Here's how the part is built. I have some questions about the finished solid (model axes, mm). A direction names the side the tool comes from. Round coordinates to 2 decimals unless told otherwise and drop trailing zeros. Write each loop counter-clockwise with the first axis right and the second up, starting at its lowest first coordinate (ties: lowest second). Pieces come first, ordered by that corner, then holes. Notation, with made-up numbers: (-30.75, -32.75) - (-12.75, -32.75) arc R6 cw to (-12.75, -21.75) - close; hole circle Ø5 at (75, -25). An arc over 180 degrees is marked (long way). Write item = value, one per line. Start each with the question number.
Item 1: If I drill on line 1 along Z through (x, y) = (54.75, -17.5); line 2 along Z through (x, y) = (-65, -22); line 3 along X through (y, z) = (-39.5, 45), over which ranges is the centre line in solid material (lowest first)? Write a range as [from, to].
Item 2: Which directions (+Z, -Z, +X, -X, +Y, -Y) give clear straight access to the entire face, cutting with the end or side of a thin tool? Please do faces 1 (the face through (-9.764, -44.614, 74.362)), 2 (the face through (79.26, -7.96, 23)), 3 (the face through (65.651, -17.745, 60.043)).
Item 3: Thinking about a two-plate mould opening in Y: for faces 4 (the face through (-1, 0, 1)), 5 (the face through (-75.72, -17.74, -75.49)), 6 (the face through (69.38, -18.58, 15.12)), which applies, pulls with the +Y half, pulls with the -Y half, needs draft (parallel to the pull), parting line crosses it, or undercut?
Item 4: For P1, Ø1, axis at y = -46, z = 43.5, coming from the -X side; P2, Ø16, axis at y = -17.5, z = 20, coming from the +X side; P3, Ø3, axis at x = 60, z = -55.5, coming from the -Y side, each with a flat end and sliding along its axis, tell me the tip position at first contact or that it passes through.
Item 5: If we section it at A-A (y = -51.5): Please give me the cut outline in (x, z).
```python
from build123d import *

# Parameters (mm, degrees)
F0_W      = 160
F0_H      = 160
F0_R      = 75
F1_DEPTH  = 35
F2_DEPTH  = 57.5
F3_SIZE2  = 3
F3_SIZE   = 3
F4_R      = 15
F5_D      = 10
F7_D      = 8
F7_DEPTH  = 40
F8_R      = 4
F9_DEPTH  = 34.5
F8_R_2    = 5
F10_DEPTH = 20
F8_R_3    = 10
F11_DEPTH = 1.5


with BuildPart() as f1:
    # F0 (on Front) → F1 (new body)
    with BuildSketch(Plane.XZ):
        Rectangle(F0_W, F0_H)
        Circle(F0_R, mode=Mode.SUBTRACT)
        Circle(F0_R)
    extrude(amount=F1_DEPTH)

    # F0 (on Front) → F2 (join)
    with BuildSketch(Plane.XZ):
        Circle(F0_R)
    extrude(amount=F2_DEPTH)

    # F3
    f3_edges = [f1.edges().sort_by_distance(p)[0] for p in [
        (-75, -57.5, 0),
    ]]
    chamfer(f3_edges, length=F3_SIZE, length2=F3_SIZE2)

    # F4
    f4_edges = [f1.edges().sort_by_distance(p)[0] for p in [
        (-80, -17.5, 80),
        (-80, -17.5, -80),
        (80, -17.5, -80),
        (80, -17.5, 80),
    ]]
    fillet(f4_edges, radius=F4_R)

    # F5 (through all)
    with Locations(Plane(origin=(0, 0, 0), x_dir=(1, 0, 0), z_dir=(0, 1, 0))):
        with Locations((-65, 65), (65, 65), (65, -65), (-65, -65)):
            Hole(F5_D / 2)

    # F7
    with Locations(Plane.XZ.offset(57.5)):
        with Locations((50, 20)):
            Hole(F7_D / 2, depth=F7_DEPTH)

    # F8 (on face) → F9 (cut)
    with BuildSketch(Plane.YZ.offset(80)):
        with Locations((-17.5, 20)):
            Circle(F8_R)
    extrude(amount=-F9_DEPTH, mode=Mode.SUBTRACT)

    # F8 (on face) → F10 (cut)
    with BuildSketch(Plane.YZ.offset(80)):
        with Locations((-17.5, 20)):
            Circle(F8_R_2)
        with Locations((-17.5, 20)):
            Circle(F8_R, mode=Mode.SUBTRACT)
    extrude(amount=-F10_DEPTH, mode=Mode.SUBTRACT)

    # F8 (on face) → F11 (cut)
    with BuildSketch(Plane.YZ.offset(80)):
        with Locations((-17.5, 20)):
            Circle(F8_R_3)
        with Locations((-17.5, 20)):
            Circle(F8_R_2, mode=Mode.SUBTRACT)
    extrude(amount=-F11_DEPTH, mode=Mode.SUBTRACT)


solid = f1.part
```
Reply:
q1.line_1 = [-80, 16], [24, 80]
q1.line_2 = [-80, -70], [-60, 60], [70, 80]
q1.line_3 = [-60, 60]
q2.face_1 = -Y
q2.face_2 = +X
q2.face_3 = +Y, -Y
q3.face_4 = pulls with the +Y half
q3.face_5 = needs draft
q3.face_6 = undercut
q4.P1 = -61.45
q4.P2 = 78.5
q4.P3 = -35
q5.outline = circle Ø150 at (0, 0); hole circle Ø8 at (50, 20)
